Drawing for the job (mm, zero at the part's lowest x, y, z). Round coordinates to 2 decimals unless told otherwise and drop trailing zeros. Write each loop counter-clockwise with the first axis right and the second up, starting at its lowest first coordinate (ties: lowest second). Pieces come first, ordered by that corner, then holes.
Item 1: Wall check: probe 1 along Y at (x, z) = (3.6, 2.3); probe 2 along X at (y, z) = (2.25, 3.1); probe 3 along Y at (x, z) = (5.2, 3.5). Give the ranges that are in metal, low to high.
Item 2: Band-saw the part on B-B, the plane z = 4.2. Write the cut outline in (x, y).
Item 3: Mould opens along Z. For the marked faces 1, 2 and 3 say: +Z half, -Z half, draft (parallel to the pull), parting line (faces both ways), or undercut.
Item 4: Band-saw the part on A-A, the plane x = 2.5. Write the cut outline in (y, z) (1 decimal).
Item 5: Drop flat-ended pins along their axis: pin 1 Ø3 at (x, y) = (1.5, 5) entering from -Z; pin 2 Ø1 at (y, z) = (5, 4.5) entering from +X. Give the stop position or say it passes through.
Item 6: Band-saw the part on D-D, the plane z = 5.65. Write the cut outline in (x, y).
Item 7: Band-saw the part on C-C, the plane y = 1.5. Write the cut outline in (x, z).
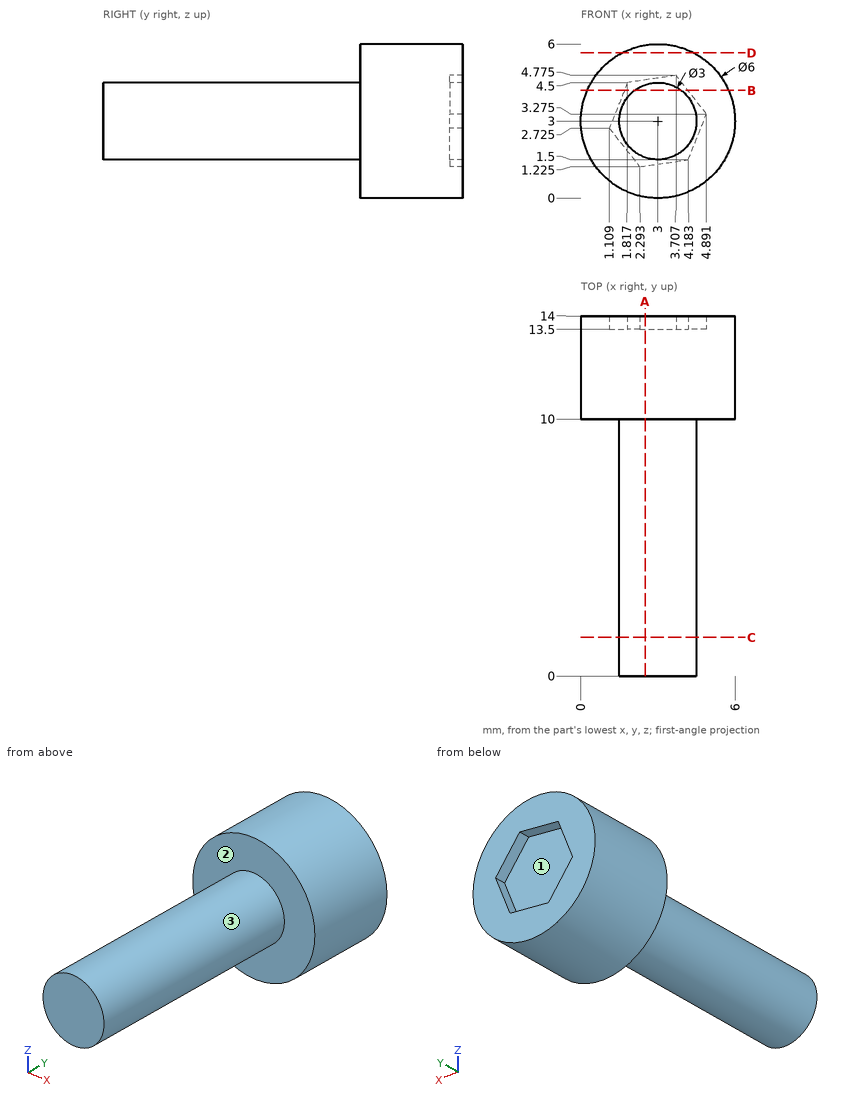
Results:
1. probe 1: y = 0 to 13.5
1. probe 2: x = 1.5 to 4.5
1. probe 3: y = 10 to 14
2. outline: (0.25, 10) - (2.1, 10) - (2.1, 0) - (3.9, 0) - (3.9, 10) - (5.75, 10) - (5.75, 14) - (4.16, 14) - (4.16, 13.5) - (1.7, 13.5) - (1.7, 14) - (0.25, 14) - close
3. face 1: undercut
3. face 2: draft
3. face 3: parting line
4. outline: (0, 1.6) - (10, 1.6) - (10, 0) - (14, 0) - (14, 1.3) - (13.5, 1.3) - (13.5, 4.6) - (14, 4.6) - (14, 6) - (10, 6) - (10, 4.4) - (0, 4.4) - close
5. pin 1: stops at z = 1.5
5. pin 2: stops at x = 4.12
6. outline: (1.59, 10) - (4.41, 10) - (4.41, 14) - (1.59, 14) - close
7. outline: circle Ø3 at (3, 3)
